```python
from build123d import *

# Parameters (mm, degrees)
F1_DEPTH = 28
F2_W     = 10
F2_H     = 18
F3_DEPTH = 2.5
F2_R     = 1.4
F4_DEPTH = 25


with BuildPart() as f1:
    # F0 (on Top) → F1 (new body)
    with BuildSketch(Plane.XY):
        Polygon((0, 7), (0, 0), (10, 0), (10, 7), (7.5, 10), (2.5, 10), align=None)
    extrude(amount=F1_DEPTH)

    # F2 (on face) → F3 (cut)
    with BuildSketch(Plane.XZ):
        with Locations((5, 14)):
            Rectangle(F2_W, F2_H)
    extrude(amount=-F3_DEPTH, mode=Mode.SUBTRACT)

    # F2 (on face) → F4 (cut)
    with BuildSketch(Plane.XZ):
        with Locations((5, 25.5)):
            Circle(F2_R)
        with Locations((5, 2.5)):
            Circle(F2_R)
    extrude(amount=-F4_DEPTH, mode=Mode.SUBTRACT)


solid = f1.part
```
Geometry check sheet. Reference: the model listing, model coordinates, mm. A direction names the side the tool comes from. Coordinates: 2 decimals unless noted, no trailing zeros. Write each loop counter-clockwise with the first axis right and the second up, starting at its lowest first coordinate (ties: lowest second). Pieces come first, ordered by that corner, then holes. Notation, with made-up numbers: M -24.5,-25 L 4.5,-25 A26 ccw 4.5,-7 Z; hole C -38,74.25 d2. An arc over 180 degrees is marked long. Answer as a JSON object with one key per item and string values.
1. Draft check along Z on faces 1 (the cylindrical face through (5.65, 4.93, 1.26)), 2 (the flat face through (5, 5, 28)), 3 (the flat face through (10, 4, 14)). Enter one of: released by +Z, released by -Z, zero draft, split by the parting line, or undercut.
Answers below:
{"face 1": "undercut", "face 2": "released by +Z", "face 3": "zero draft"}
2. Section check D-D, the plane y = 3.25. Enter the section's corners in (x, z).
Answers below:
{"outline": "M 0,0 L 10,0 L 10,28 L 0,28 Z; hole C 5,2.5 d2.8; hole C 5,25.5 d2.8"}
3. Section check C-C, the plane z = 25.5. Enter the section's corners in (x, y), plus the area to 3 significant figures.
Answers below:
{"outline": "M 0,0 L 3.6,0 L 3.6,10 L 2.5,10 L 0,7 Z; M 6.4,0 L 10,0 L 10,7 L 7.5,10 L 6.4,10 Z", "area": "64.5 mm²"}
4. Go/stop test with a flat-tipped pin: pin 1 Ø1 at (x, z) = (3, 21) entering from -Y. Record where the tip stops, or that it passes through.
Answers below:
{"pin 1": "stops at y = 2.5"}
5. Section check B-B, the plane x = 5. Enter the section's corners in (y, z), plus the area to 3 significant figures.
Answers below:
{"outline": "M 0,0 L 10,0 L 10,1.1 L 0,1.1 Z; M 0,3.9 L 10,3.9 L 10,24.1 L 0,24.1 L 0,23 L 2.5,23 L 2.5,5 L 0,5 Z; M 0,26.9 L 10,26.9 L 10,28 L 0,28 Z", "area": "179 mm²"}
6. Section check A-A, the plane y = 1. Enter the section's corners in (x, z).
Answers below:
{"outline": "M 0,0 L 10,0 L 10,5 L 0,5 Z; M 0,23 L 10,23 L 10,28 L 0,28 Z; hole C 5,2.5 d2.8; hole C 5,25.5 d2.8"}
7. Scan lines: L1, parallel to Z at x = 5, y = 6.25; L2, parallel to Z at x = 5.5, y = 7.75; L3, parallel to Y at x = 3.25, z = 10.5. Record each from-to range of solid material in increasing order.
Answers below:
{"L1": "z = 0 to 1.1, 3.9 to 24.1, 26.9 to 28", "L2": "z = 0 to 1.19, 3.81 to 24.19, 26.81 to 28", "L3": "y = 2.5 to 10"}
8. Tool access check on faces 4 (the flat face through (6, 0, 1)), 5 (the flat face through (5, 1, 23)). Record the directions out of +Z, -Z, +X, -X, +Y, -Y that give a thin tool (end or side, any length) a straight path to the whole face; none if there is none.
Answers below:
{"face 4": "+Z, -Z, +X, -X, -Y", "face 5": "+X, -X, -Y"}
